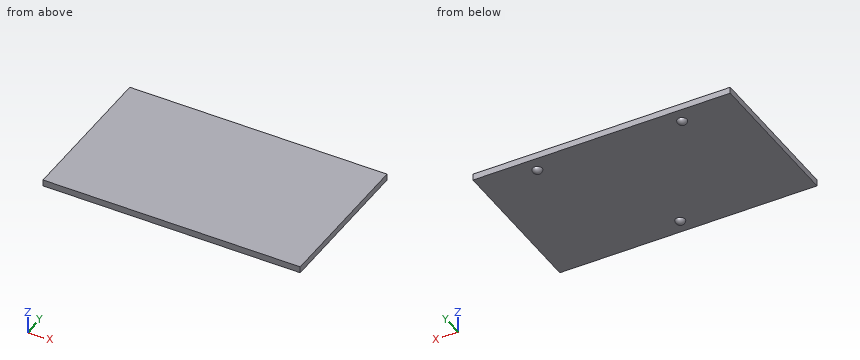
from build123d import *

# Parameters (mm, degrees)
F0_W            = 254
F0_H            = 152.4
F1_DEPTH        = 6.35
F5_COPIES_COUNT = 3


# Not quite as in the source:
# - a pattern or mirror of a feature is missing from the dataset's text; its kind, count and spacing are read off the source's solid


with BuildPart() as f1:
    # F0 (on Top) → F1 (new body)
    with BuildSketch(Plane.XY):
        Rectangle(F0_W, F0_H)
    extrude(amount=F1_DEPTH)

    # F4 (on face) → F5 (revolve)
    with BuildSketch(Plane.XZ.offset(-61.9125)):
        with BuildLine():
            Line((-71.4903970824, 0.7803010637), (-71.4903970824, -4.0456989363))
            ThreePointArc((-71.4903970824, -4.0456989363), (-68.0778997564, -2.6321962623), (-66.6643970824, 0.7803010637))
            Line((-66.6643970824, 0.7803010637), (-71.4903970824, 0.7803010637))
        make_face()
    f5 = revolve(axis=Axis((-71.4903970824, 61.9125, -1.6326989363), (0, 0, 1)))

    # F5_copies: F5 ×3 about axis
    f5_copies_axis = Axis((0, 20.6375, 0), (0, 0, 1))
    for i in range(1, F5_COPIES_COUNT):
        add(f5.rotate(f5_copies_axis, i * 360 / F5_COPIES_COUNT))


solid = f1.part
The listing builds one solid part. Answer for the finished solid, in the listing's coordinates (mm). Give positions to 0.01 mm unless a question says otherwise; leave off trailing zeros. Write each loop counter-clockwise with the first axis right and the second up, starting at its lowest first coordinate (ties: lowest second). Pieces come first, ordered by that corner, then holes.
Item 1: Section A-A, the plane y = -35 is taken. Write down the section's boundary in (x, z), plus the area to 3 significant figures.
Item 2: Find the intervals of material crossed by line 1 along Z through (x, y) = (-91.5, -14.5); line 2 along Y through (x, z) = (72, -1.5); line 3 along X through (y, z) = (62, -2.5), in increasing order.
Item 3: Flat-ended cylindrical pins translate along their axes: P1, Ø3, axis at y = 60.5, z = -3, coming from the +X side; P2, Ø5, axis at x = 42, y = 46, coming from the -Z side. Find the tip coordinate at first contact, or state that the pin passes through.
Item 4: Section B-B, the plane x = 98 is taken. Write down the section's boundary in (y, z), plus the area to 3 significant figures.
Completed:
1. outline: (-127, 0) - (127, 0) - (127, 6.35) - (-127, 6.35) - close
1. area: 1,610 mm2
2. line 1: z = 0 to 6.35
2. line 2: y = 57.69 to 66.14
2. line 3: x = -75.03 to -67.95, 67.95 to 75.03
3. P1: stops at x = 75.6
3. P2: stops at z = 0
4. outline: (-76.2, 0) - (76.2, 0) - (76.2, 6.35) - (-76.2, 6.35) - close
4. area: 968 mm2
